CAD build for the part. Positions are in the model's coordinates, mm. Face numbers are marked on the shaded views. A direction names the side the tool comes from. Give positions to 0.01 mm unless a question says otherwise; leave off trailing zeros. Loops run counter-clockwise (first coordinate to the right, second up) from the corner with the lowest first, then second, coordinate; pieces in that order, holes last. Notation, with made-up numbers: M 29,22.25 L 64,22.25 A31 ccw 64,48.25 Z; hole C 60,12 d8. An arc over 180 degrees is marked long. Answer as CSV lines item,"result".
from build123d import *

# Parameters (mm, degrees)
SKETCH1_W             = 24
SKETCH1_H             = 8
SKETCH1_R             = 1
BOSS_EXTRUDE1_DEPTH   = 5
BOSS_EXTRUDE1_2_DEPTH = 5
SKETCH2_W             = 24
SKETCH2_H             = 8
SKETCH2_R             = 1
BOSS_EXTRUDE2_DEPTH   = 8
BOSS_EXTRUDE3_DEPTH   = 10
CHAMFER1_SIZE         = 1
FILLET1_R             = 2
SKETCH3_R             = 1
CUT_EXTRUDE1_DEPTH    = 7


with BuildPart() as part:
    # Sketch1 → Boss-Extrude1 (new body)
    with BuildSketch(Plane.XY):
        with Locations((-8.500045519, -6.479626746)):
            Rectangle(SKETCH1_W, SKETCH1_H)
        with Locations(Location((0.499954481, -6.479626746, 0), (0, 0, 180))):
            Circle(SKETCH1_R, mode=Mode.SUBTRACT)
        with Locations((-14.500045519, -4.479626746)):
            Circle(SKETCH1_R, mode=Mode.SUBTRACT)
        with Locations((-2.500045519, -8.479626746)):
            Circle(SKETCH1_R, mode=Mode.SUBTRACT)
        with Locations((-17.500045519, -6.479626746)):
            Circle(SKETCH1_R, mode=Mode.SUBTRACT)
        with Locations(Location((-14.500045519, -8.479626746, 0), (0, 0, 180))):
            Circle(SKETCH1_R, mode=Mode.SUBTRACT)
        with Locations(Location((-2.500045519, -4.479626746, 0), (0, 0, 180))):
            Circle(SKETCH1_R, mode=Mode.SUBTRACT)
    extrude(amount=BOSS_EXTRUDE1_DEPTH)



with BuildPart() as body_2:
    # Sketch1 → Boss-Extrude1 2 (new body)
    with BuildSketch(Plane.XY):
        with Locations((16.499954481, 6.520373254)):
            Rectangle(SKETCH1_W, SKETCH1_H)
        with Locations((10.499954481, 8.520373254)):
            Circle(SKETCH1_R, mode=Mode.SUBTRACT)
        with Locations((7.499954481, 6.520373254)):
            Circle(SKETCH1_R, mode=Mode.SUBTRACT)
        with Locations(Location((10.499954481, 4.520373254, 0), (0, 0, 180))):
            Circle(SKETCH1_R, mode=Mode.SUBTRACT)
        with Locations((22.499954481, 4.520373254)):
            Circle(SKETCH1_R, mode=Mode.SUBTRACT)
        with Locations(Location((25.499954481, 6.520373254, 0), (0, 0, 180))):
            Circle(SKETCH1_R, mode=Mode.SUBTRACT)
        with Locations(Location((22.499954481, 8.520373254, 0), (0, 0, 180))):
            Circle(SKETCH1_R, mode=Mode.SUBTRACT)
    extrude(amount=BOSS_EXTRUDE1_2_DEPTH)


with BuildPart() as part_1:
    add(part.part)

    add(body_2.part)  # Boss-Extrude2 merges body 2
    # Sketch2 → Boss-Extrude2 (add)
    # profile 1 of 3: a face of its own
    with BuildSketch(Plane.XY.offset(5)):
        with Locations((-8.500045519, -6.479626746)):
            Rectangle(SKETCH2_W, SKETCH2_H)
        with Locations(Location((-14.500045519, -8.479626746, 0), (0, 0, 180))):
            Circle(SKETCH2_R, mode=Mode.SUBTRACT)
        with Locations((-17.500045519, -6.479626746)):
            Circle(SKETCH2_R, mode=Mode.SUBTRACT)
        with Locations((-2.500045519, -8.479626746)):
            Circle(SKETCH2_R, mode=Mode.SUBTRACT)
        with Locations(Location((0.499954481, -6.479626746, 0), (0, 0, 180))):
            Circle(SKETCH2_R, mode=Mode.SUBTRACT)
        with Locations((-14.500045519, -4.479626746)):
            Circle(SKETCH2_R, mode=Mode.SUBTRACT)
        with Locations(Location((-2.500045519, -4.479626746, 0), (0, 0, 180))):
            Circle(SKETCH2_R, mode=Mode.SUBTRACT)
    # profile 2 of 3: a face of its own
    with BuildSketch(Plane.XY.offset(5)):
        Polygon((3.499954481, -2.479626746), (3.499954481, -10.479626746), (28.499954481, -10.479626746), (28.499954481, 2.520373254), (4.499954481, 2.520373254), (4.499954481, 10.520373254), (-20.500045519, 10.520373254), (-20.500045519, -2.479626746), align=None)
    # profile 3 of 3: a face of its own
    with BuildSketch(Plane.XY.offset(5)):
        with Locations((16.499954481, 6.520373254)):
            Rectangle(SKETCH2_W, SKETCH2_H)
        with Locations(Location((10.499954481, 4.520373254, 0), (0, 0, 180))):
            Circle(SKETCH2_R, mode=Mode.SUBTRACT)
        with Locations((22.499954481, 4.520373254)):
            Circle(SKETCH2_R, mode=Mode.SUBTRACT)
        with Locations((7.499954481, 6.520373254)):
            Circle(SKETCH2_R, mode=Mode.SUBTRACT)
        with Locations((10.499954481, 8.520373254)):
            Circle(SKETCH2_R, mode=Mode.SUBTRACT)
        with Locations(Location((25.499954481, 6.520373254, 0), (0, 0, 180))):
            Circle(SKETCH2_R, mode=Mode.SUBTRACT)
        with Locations(Location((22.499954481, 8.520373254, 0), (0, 0, 180))):
            Circle(SKETCH2_R, mode=Mode.SUBTRACT)
    extrude(amount=BOSS_EXTRUDE2_DEPTH)

    # Sketch2<6> → Boss-Extrude3 (add)
    with BuildSketch(Plane.XY.offset(5)):
        Polygon((3.499954481, -2.479626746), (3.499954481, -10.479626746), (28.499954481, -10.479626746), (28.499954481, 2.520373254), (4.499954481, 2.520373254), (4.499954481, 10.520373254), (-20.500045519, 10.520373254), (-20.500045519, -2.479626746), align=None)
    extrude(amount=BOSS_EXTRUDE3_DEPTH)

    # Chamfer1
    # the kernel refuses this chamfer: 1 mm, written as the material it takes off along each edge
    with BuildSketch(Plane(origin=(25.499954481, 6.520373254, 13), x_dir=(-1, 0, 0), z_dir=(0, 1, 0))) as chamfer1_piece_1:
        Polygon((1 + CHAMFER1_SIZE, 0), (1, -CHAMFER1_SIZE), (1, 0), align=None)
    revolve(axis=Axis((25.499954481, 6.520373254, 13), (0, 0, 1)), mode=Mode.SUBTRACT)
    with BuildSketch(Plane(origin=(22.499954481, 8.520373254, 13), x_dir=(-1, 0, 0), z_dir=(0, 1, 0))) as chamfer1_piece_2:
        Polygon((1 + CHAMFER1_SIZE, 0), (1, -CHAMFER1_SIZE), (1, 0), align=None)
    revolve(axis=Axis((22.499954481, 8.520373254, 13), (0, 0, 1)), mode=Mode.SUBTRACT)
    with BuildSketch(Plane(origin=(10.499954481, 4.520373254, 13), x_dir=(-1, 0, 0), z_dir=(0, 1, 0))) as chamfer1_piece_3_section:
        Polygon((1 + CHAMFER1_SIZE, 0), (1, -CHAMFER1_SIZE), (1, 0), align=None)
    chamfer1_piece_3 = revolve(axis=Axis((10.499954481, 4.520373254, 13), (0, 0, 1)), mode=Mode.PRIVATE)
    chamfer1_piece_3 = split(chamfer1_piece_3, bisect_by=Plane(origin=(11.988197193, 2.520373254, 12.511757288), z_dir=(0, 1, 0)), keep=Keep.TOP, mode=Mode.PRIVATE)
    add(chamfer1_piece_3, mode=Mode.SUBTRACT)
    with BuildSketch(Plane(origin=(10.499954481, 8.520373254, 13), x_dir=(1, 0, 0), z_dir=(0, -1, 0))) as chamfer1_piece_4:
        Polygon((1 + CHAMFER1_SIZE, 0), (1, -CHAMFER1_SIZE), (1, 0), align=None)
    revolve(axis=Axis((10.499954481, 8.520373254, 13), (0, 0, 1)), mode=Mode.SUBTRACT)
    with BuildSketch(Plane(origin=(7.499954481, 6.520373254, 13), x_dir=(1, 0, 0), z_dir=(0, -1, 0))) as chamfer1_piece_5:
        Polygon((1 + CHAMFER1_SIZE, 0), (1, -CHAMFER1_SIZE), (1, 0), align=None)
    revolve(axis=Axis((7.499954481, 6.520373254, 13), (0, 0, 1)), mode=Mode.SUBTRACT)
    with BuildSketch(Plane(origin=(22.499954481, 4.520373254, 13), x_dir=(1, 0, 0), z_dir=(0, -1, 0))) as chamfer1_piece_6_section:
        Polygon((1 + CHAMFER1_SIZE, 0), (1, -CHAMFER1_SIZE), (1, 0), align=None)
    chamfer1_piece_6 = revolve(axis=Axis((22.499954481, 4.520373254, 13), (0, 0, 1)), mode=Mode.PRIVATE)
    chamfer1_piece_6 = split(chamfer1_piece_6, bisect_by=Plane(origin=(21.011711773, 2.520373254, 12.511757292), z_dir=(0, 1, 0)), keep=Keep.TOP, mode=Mode.PRIVATE)
    add(chamfer1_piece_6, mode=Mode.SUBTRACT)
    with BuildSketch(Plane(origin=(-14.500045519, -8.479626746, 13), x_dir=(-1, 0, 0), z_dir=(0, 1, 0))) as chamfer1_piece_7:
        Polygon((1 + CHAMFER1_SIZE, 0), (1, -CHAMFER1_SIZE), (1, 0), align=None)
    revolve(axis=Axis((-14.500045519, -8.479626746, 13), (0, 0, 1)), mode=Mode.SUBTRACT)
    with BuildSketch(Plane(origin=(-2.500045519, -8.479626746, 13), x_dir=(1, 0, 0), z_dir=(0, -1, 0))) as chamfer1_piece_8:
        Polygon((1 + CHAMFER1_SIZE, 0), (1, -CHAMFER1_SIZE), (1, 0), align=None)
    revolve(axis=Axis((-2.500045519, -8.479626746, 13), (0, 0, 1)), mode=Mode.SUBTRACT)
    with BuildSketch(Plane(origin=(-2.500045519, -4.479626746, 13), x_dir=(-1, 0, 0), z_dir=(0, 1, 0))) as chamfer1_piece_9_section:
        Polygon((1 + CHAMFER1_SIZE, 0), (1, -CHAMFER1_SIZE), (1, 0), align=None)
    chamfer1_piece_9 = revolve(axis=Axis((-2.500045519, -4.479626746, 13), (0, 0, 1)), mode=Mode.PRIVATE)
    chamfer1_piece_9 = split(chamfer1_piece_9, bisect_by=Plane(origin=(-1.011802811, -2.479626746, 12.511757292), z_dir=(0, -1, 0)), keep=Keep.TOP, mode=Mode.PRIVATE)
    add(chamfer1_piece_9, mode=Mode.SUBTRACT)
    with BuildSketch(Plane(origin=(-17.500045519, -6.479626746, 13), x_dir=(1, 0, 0), z_dir=(0, -1, 0))) as chamfer1_piece_10:
        Polygon((1 + CHAMFER1_SIZE, 0), (1, -CHAMFER1_SIZE), (1, 0), align=None)
    revolve(axis=Axis((-17.500045519, -6.479626746, 13), (0, 0, 1)), mode=Mode.SUBTRACT)
    with BuildSketch(Plane(origin=(-14.500045519, -4.479626746, 13), x_dir=(1, 0, 0), z_dir=(0, -1, 0))) as chamfer1_piece_11_section:
        Polygon((1 + CHAMFER1_SIZE, 0), (1, -CHAMFER1_SIZE), (1, 0), align=None)
    chamfer1_piece_11 = revolve(axis=Axis((-14.500045519, -4.479626746, 13), (0, 0, 1)), mode=Mode.PRIVATE)
    chamfer1_piece_11 = split(chamfer1_piece_11, bisect_by=Plane(origin=(-15.988288231, -2.479626746, 12.511757288), z_dir=(0, -1, 0)), keep=Keep.TOP, mode=Mode.PRIVATE)
    add(chamfer1_piece_11, mode=Mode.SUBTRACT)
    with BuildSketch(Plane(origin=(0.499954481, -6.479626746, 13), x_dir=(-1, 0, 0), z_dir=(0, 1, 0))) as chamfer1_piece_12:
        Polygon((1 + CHAMFER1_SIZE, 0), (1, -CHAMFER1_SIZE), (1, 0), align=None)
    revolve(axis=Axis((0.499954481, -6.479626746, 13), (0, 0, 1)), mode=Mode.SUBTRACT)

    # Fillet1
    fillet1_edges = [part_1.edges().sort_by_distance(p)[0] for p in [
        (28.499954481, -10.479626746, 10),
        (28.499954481, 10.520373254, 6.5),
        (-20.500045519, 10.520373254, 10),
        (-20.500045519, -10.479626746, 6.5),
    ]]
    fillet(fillet1_edges, radius=FILLET1_R)

    # Sketch3 → Cut-Extrude1 (cut)
    with BuildSketch(Plane.XY.offset(15)):
        with Locations((-16.000045519, 0.020373254)):
            Circle(SKETCH3_R)
        with Locations((-16.000045519, 5.020373254)):
            Circle(SKETCH3_R)
        with Locations((-6.000045519, 5.020373254)):
            Circle(SKETCH3_R)
        with Locations((-6.000045519, 0.020373254)):
            Circle(SKETCH3_R)
        with Locations((3.999954481, 0.020373254)):
            Circle(SKETCH3_R)
        with Locations((13.999954481, 0.020373254)):
            Circle(SKETCH3_R)
        with Locations((13.999954481, -4.979626746)):
            Circle(SKETCH3_R)
        with Locations((23.999954481, 0.020373254)):
            Circle(SKETCH3_R)
        with Locations((23.999954481, -4.979626746)):
            Circle(SKETCH3_R)
    extrude(amount=-CUT_EXTRUDE1_DEPTH, mode=Mode.SUBTRACT)


solid = part_1.part
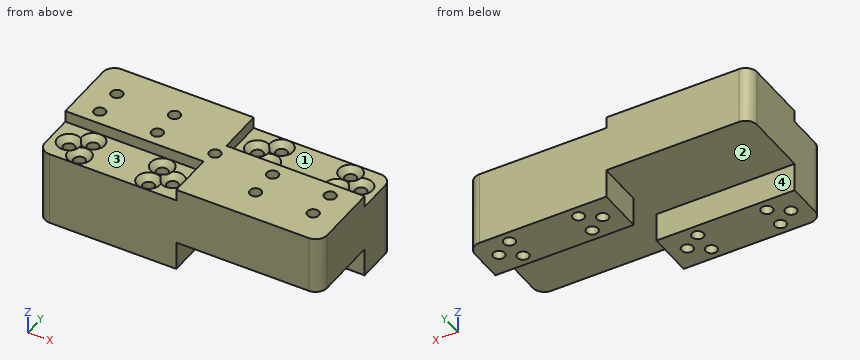
1) Band-saw the part on B-B on x = 20. Give the cut face in (y, z), and give its area (3 significant figures).
Answer below:
outline,"M -10.48,5 L 2.52,5 L 2.52,0 L 10.52,0 L 10.52,13 L 2.52,13 L 2.52,15 L -10.48,15 Z"
area,"234 mm^2"
2) Drill centre lines: line 1 (Y direction, x = -14.5, z = 2); line 2 (X direction, y = 5, z = 10.5); line 3 (X direction, y = -5, z = 11.5). Where is each one in solid material? Low to high. Write a range as from..to.
Answer below:
line 1,"y = -10.48..-9.48, -7.48..-5.48, -3.48..-2.48"
line 2,"x = -20.5..-17, -15..-7, -5..9.62, 11.38..21.62, 23.38..28.5"
line 3,"x = -20.5..-15.35, -13.65..-3.35, -1.65..13, 15..23, 25..28.5"
3) Band-saw the part on A-A on z = 2. Give the number of separate pieces and of enclosed holes in the cut face, and give its area (3 significant figures).
Answer below:
separate pieces,"2"
enclosed holes,"12"
area,"345 mm^2"
4) Which spindle directions (+Z, -Z, +X, -X, +Y, -Y) get a long thin tool onto all of the face, cutting with end or side? Do the marked faces 1, 2, 3 and 4. Say none if no direction does.
Answer below:
face 1,"+Z, +X, +Y"
face 2,"-Z"
face 3,"+Z, -X, -Y"
face 4,"-Z, +X, -X, +Y"
5) Band-saw the part on D-D on y = -2. Give the cut face in (x, z).
Answer below:
outline,"M -20.5,5 L 28.5,5 L 28.5,15 L -20.5,15 Z"
6) Flat gauge pins, fed straight in: pin 1 (2.5 mm diameter, centred on x = 25.5, y = 6.52, fed in from +Z); pin 2 (1.8 mm diameter, centred on x = -6, y = 0.02, fed in from +Z); pin 3 (1.8 mm diameter, centred on x = 7.5, y = 8, fed in from +Z). Where does each tip first touch, or does it go through?
Answer below:
pin 1,"stops at z = 12.25"
pin 2,"stops at z = 8"
pin 3,"stops at z = 13"
